```python
from build123d import *

# Parameters (mm, degrees)
CROQUIS1_W              = 10.950949918
CROQUIS1_H              = 9.461001059
CROQUIS2_R              = 4
SALIENTE_EXTRUIR1_DEPTH = 4
CORTAR_EXTRUIR1_DEPTH   = 10
MATRIZC1_COUNT          = 3
CORTAR_EXTRUIR2_START   = -7
CROQUIS8_R              = 9.607815028
CORTAR_EXTRUIR2_DEPTH   = 7
CROQUIS9_R              = 1.019703071
CORTAR_EXTRUIR3_DEPTH   = 21.519384926
ESCALA1_SCALE           = 0.565


with BuildPart() as part:
    # Croquis1 → Revolución1 (revolve)
    with BuildSketch(Plane(origin=(0, 0, 0), x_dir=(-1, 0, 0), z_dir=(0, 0, -1)), mode=Mode.PRIVATE) as revoluci_n1_sk:
        with Locations((-5.475474959, 8.73050053)):
            Rectangle(CROQUIS1_W, CROQUIS1_H)
    revolve(revoluci_n1_sk.sketch.rotate(Axis((0, 4, 0), (0, 1, 0)), 270), axis=Axis((0, 4, 0), (0, 1, 0)))

    # Croquis2 → Saliente-Extruir1 (add)
    with BuildSketch(Plane.XZ.offset(-4)):
        with Locations(Location((0, 0, 0), (0, 0, 270))):
            Circle(CROQUIS2_R)
    extrude(amount=SALIENTE_EXTRUIR1_DEPTH)

    # Croquis7 → Cortar-Extruir1 (cut)
    with BuildSketch(Plane.XZ.offset(-4)):
        with BuildLine():
            Line((2.290412928, 3.737743004), (4.394709568, 8.543806963))
            ThreePointArc((4.394709568, 8.543806963), (9.368666462, 2.13030475), (7.657065469, -5.803400555))
            Line((7.657065469, -5.803400555), (4.382944907, -0.080672706))
            ThreePointArc((4.382944907, -0.080672706), (3.844281576, 2.106706746), (2.290412928, 3.737743004))
        make_face()
    cortar_extruir1 = extrude(amount=-CORTAR_EXTRUIR1_DEPTH, mode=Mode.SUBTRACT)

    # MatrizC1: Cortar-Extruir1 ×3 about axis
    matrizc1_axis = Axis((0, 0, 0), (0, 1, 0))
    for i in range(1, MATRIZC1_COUNT):
        add(cortar_extruir1.rotate(matrizc1_axis, i * 360 / MATRIZC1_COUNT), mode=Mode.SUBTRACT)

    # Croquis8 → Cortar-Extruir2 (cut)
    with BuildSketch(Plane(origin=(0, 13.461001059, 0), x_dir=(1, 0, 0), z_dir=(0, 1, 0)).offset(CORTAR_EXTRUIR2_START)):
        with Locations(Location((0, 0, 0), (0, 0, 57.220098004))):
            Circle(CROQUIS8_R)
    extrude(amount=CORTAR_EXTRUIR2_DEPTH, mode=Mode.SUBTRACT)

    # Croquis9 → Cortar-Extruir3 (cut, through all)
    with BuildSketch(Plane.XZ):
        with Locations(Location((0, 0, 0), (0, 0, 270))):
            Circle(CROQUIS9_R)
    extrude(amount=-CORTAR_EXTRUIR3_DEPTH, mode=Mode.SUBTRACT)


with BuildPart() as part_1:
    # Escala1: scaled about (0, 6.977093027, 0)
    add(part.part.scale(ESCALA1_SCALE).moved(Location((0, 3.035035467, 0))))


solid = part_1.part
```
Can you work these out from the model? Positions are in its coordinate system, mm. A direction names the side the tool comes from. Coordinates: 2 decimals unless noted, no trailing zeros. Loops run counter-clockwise (first coordinate to the right, second up) from the corner with the lowest first, then second, coordinate; pieces in that order, holes last. Notation, with made-up numbers: (78, 30) - (102, 30) arc R12 cw to (102, 40) - close; hole circle Ø5 at (-17.5, 14). An arc over 180 degrees is marked (long way). Answer as CSV lines item,"result". Start each with the question number.
1) Suppose I cut it at C-C (x = 3.75). Please give me the cut outline in (y, z).
2) Suppose I cut it at A-A (y = 6). Please give me the cut outline in (x, z).
3) For pin 1 (3 mm diameter, centred on x = 2, z = 2.5, fed in from +Y); pin 2 (2 mm diameter, centred on x = 3.5, z = 4.5, fed in from -Y); pin 3 (0.7 mm diameter, centred on x = 0, z = 0, fed in from -Y), each with a flat end and sliding along its axis, tell me the tip position at first contact or that it passes through.
4) Suppose I cut it at D-D (y = 8). Please give me the cut outline in (x, z).
5) Suppose I cut it at B-B (z = 0.25). Please give me the cut outline in (x, y), plus the area to 3 significant figures.
6) I need wall thicknesses on line 1 (X direction, y = 4.4, z = 0); line 2 (Z direction, x = -1, y = 6.25); line 3 (Z direction, x = -4.75, y = 5.5). Which ranges of each line are inside material? Lowest first, please. Write a range as from..to.
7) Thinking about a two-plate mould opening in Z: for faces 1 (the cylindrical face through (5.217, 8.005, 3.326)), 2 (the cylindrical face through (2.181, 5.981, 1.174)), 3 (the flat face through (1, 3.035, 0)), which applies, pulls with the +Z half, pulls with the -Z half, needs draft (parallel to the pull), parting line crosses it, or undercut?
8) Which directions (+Z, -Z, +X, -X, +Y, -Y) give clear straight access to the entire face, cutting with the end or side of a thin tool? Please do faces 4 (the flat face through (1, 6.686, 0)), 5 (the flat face through (-4, 10.641, 4)), 6 (the cylindrical face through (0.679, 4.181, -2.156)), 7 (the cylindrical face through (-2.11, 5.98, 1.3)).
Check result:
1,outline,"(5.3, -4.92) - (10.64, -4.92) - (10.64, -3.92) - (6.69, -3.92) - (6.69, -2.27) - (5.3, -2.27) - close; (5.3, 3.92) - (10.64, 3.92) - (10.64, 4.92) - (5.3, 4.92) - close"
2,outline,"circle Ø12.37 at (0, 0); hole (-5.42, -0.26) - (-2.48, 0.06) arc R2.48 cw to (-1.2, 2.17) - (0.68, 5.39) arc R5.43 ccw to start; hole (-5, -2.11) arc R5.43 ccw to (2.94, -4.56) - (1.18, -2.18) arc R2.48 cw to (-1.28, -2.12) - close; hole circle Ø1.15 at (0, 0); hole (1.29, 2.11) arc R2.48 cw to (2.48, -0.05) - (4.33, -3.28) arc R5.43 ccw to (2.48, 4.83) - close"
3,pin 1,"stops at y = 6.69"
3,pin 2,"stops at y = 5.3"
3,pin 3,"passes through"
4,outline,"circle Ø12.37 at (0, 0); hole circle Ø10.86 at (0, 0)"
5,outline,"(-6.18, 5.3) - (-5.42, 5.3) - (-5.42, 10.64) - (-6.18, 10.64) - close; (-2.46, 5.3) - (-2.25, 5.3) - (-2.25, 3.04) - (-0.52, 3.04) - (-0.52, 6.69) - (-2.46, 6.69) - close; (0.52, 3.04) - (2.25, 3.04) - (2.25, 5.3) - (2.46, 5.3) - (2.46, 6.69) - (0.52, 6.69) - close; (5.42, 5.3) - (6.18, 5.3) - (6.18, 10.64) - (5.42, 10.64) - close"
5,area,"21.3 mm²"
6,line 1,"x = -2.26..-0.58, 0.58..2.26"
6,line 2,"z = -6.11..-5.34, -2.27..2.51, 5.34..6.11"
6,line 3,"z = -3.96..-2.63, -2.11..-0.19, 2.63..3.96"
7,face 1,"parting line crosses it"
7,face 2,"undercut"
7,face 3,"needs draft"
8,face 4,"+Y"
8,face 5,"+Z, -Z, +X, -X, +Y"
8,face 6,"-Y"
8,face 7,"+Y, -Y"
